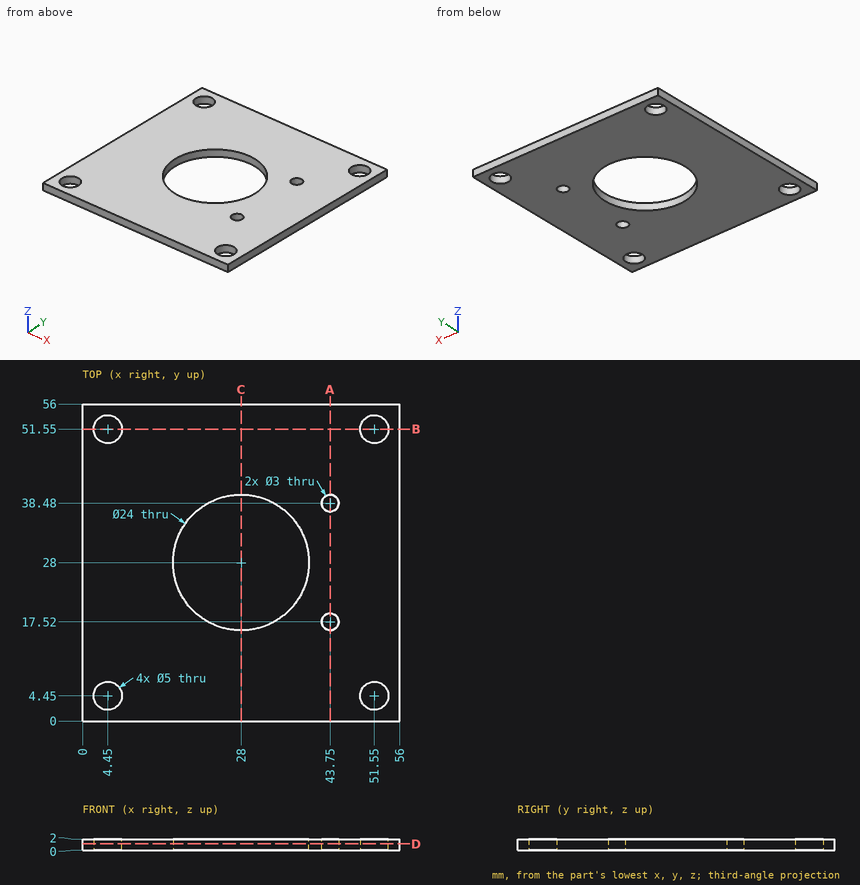
Verification items for this drawing (mm, ordinates from the low corner). Give positions to 0.01 mm unless a question says otherwise; leave off trailing zeros. Write each loop counter-clockwise with the first axis right and the second up, starting at its lowest first coordinate (ties: lowest second). Pieces come first, ordered by that corner, then holes. Notation, with made-up numbers: (-28.75, 1) - (4.25, 1) arc R8 ccw to (4.25, 6) - close; hole circle Ø11 at (74, 43.5). An arc over 180 degrees is marked (long way). Answer as a JSON object with one key per item and string values. Group by question number.
1) Sectioned sample at B-B (y = 51.55). Record the cut outline in (x, z), then the cut area to 3 significant figures.
2) Sectioned sample at D-D (z = 1.15). Record the cut outline in (x, y).
3) Thickness scan on probe 1 along X at (y, z) = (51.55, 0.4); probe 2 along Y at (x, z) = (43.75, 1.3). Record the ranges inside material, lowest first. Write a range as from..to.
4) Sectioned sample at C-C (x = 28). Record the cut outline in (y, z).
5) Sectioned sample at A-A (x = 43.75). Record the cut outline in (y, z), then the cut area to 3 significant figures.
6) Depth check by flat-ended pin: P1, Ø21.5, axis at x = 28, y = 28, coming from the -Z side (1 decimal). Enter the tip coordinate at first touch or a pass-through.
Geometry results:
{
 "1": {"outline": "(0, 0) - (1.95, 0) - (1.95, 2) - (0, 2) - close; (6.95, 0) - (49.05, 0) - (49.05, 2) - (6.95, 2) - close; (54.05, 0) - (56, 0) - (56, 2) - (54.05, 2) - close", "area": "92.0 mm^2"},
 "2": {"outline": "(0, 0) - (56, 0) - (56, 56) - (0, 56) - close; hole circle Ø5 at (4.45, 4.45); hole circle Ø5 at (4.45, 51.55); hole circle Ø24 at (28, 28); hole circle Ø3 at (43.75, 17.52); hole circle Ø3 at (43.75, 38.48); hole circle Ø5 at (51.55, 4.45); hole circle Ø5 at (51.55, 51.55)"},
 "3": {"probe 1": "x = 0..1.95, 6.95..49.05, 54.05..56", "probe 2": "y = 0..16.02, 19.02..36.98, 39.98..56"},
 "4": {"outline": "(0, 0) - (16, 0) - (16, 2) - (0, 2) - close; (40, 0) - (56, 0) - (56, 2) - (40, 2) - close"},
 "5": {"outline": "(0, 0) - (16.02, 0) - (16.02, 2) - (0, 2) - close; (19.02, 0) - (36.98, 0) - (36.98, 2) - (19.02, 2) - close; (39.98, 0) - (56, 0) - (56, 2) - (39.98, 2) - close", "area": "100 mm^2"},
 "6": {"P1": "passes through"}
}
